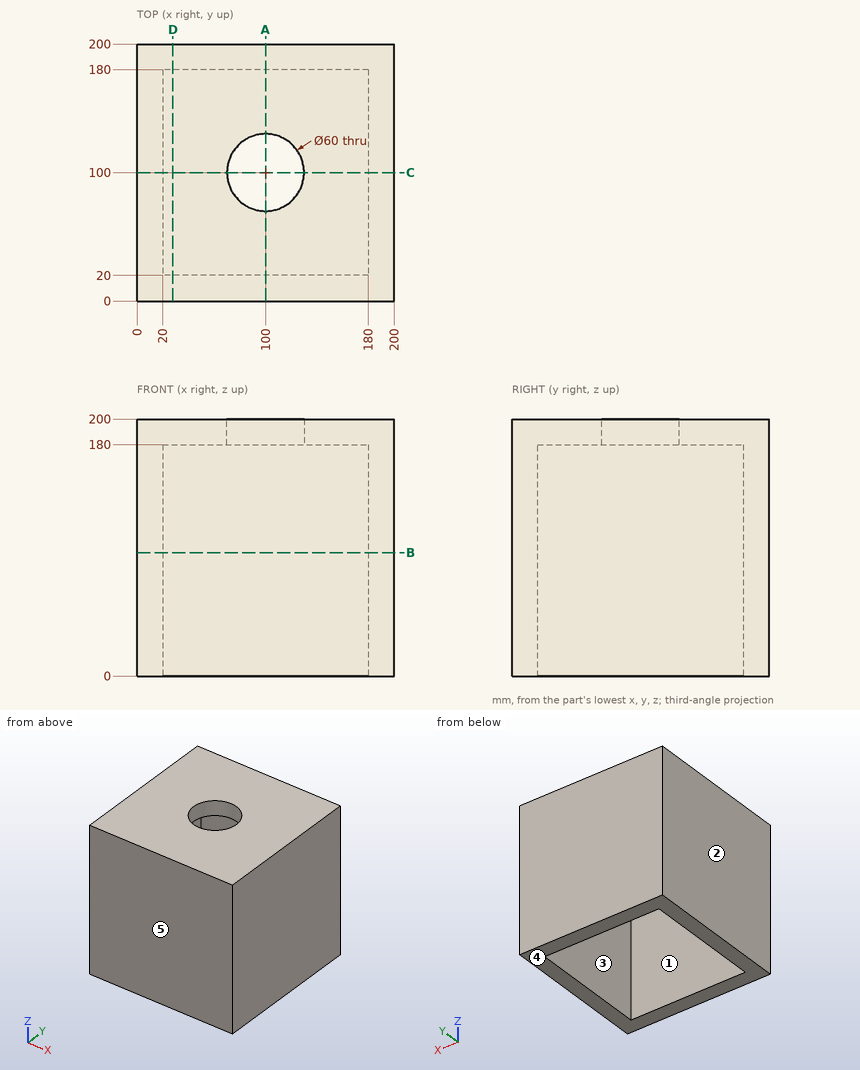
Design review of the part shown in the three views and the two pictorial views. Dimensions are in mm from the part's minimum x, y and z. A direction names the side the tool comes from. Give positions to 0.01 mm unless a question says otherwise; leave off trailing zeros. Write each loop counter-clockwise with the first axis right and the second up, starting at its lowest first coordinate (ties: lowest second). Pieces come first, ordered by that corner, then holes. Notation, with made-up numbers: (-17.75, -18) -> (4.25, -18) arc R27 cw to (4.25, 11) -> close; hole circle Ø8 at (71, 40.5). An arc over 180 degrees is marked (long way). Answer in a Markdown table with one row per item.
1) Clearance check with flat-ended pins moving along their axes: P1, Ø12, axis at x = 78, z = 85.5, coming from the -Y side; P2, Ø1, axis at x = 36.5, y = 177, coming from the -Z side. State where each tip first meets the part, or that it passes through.
Worked answers:
| item | result |
|---|---|
| P1 | y = 0 |
| P2 | z = 180 |
2) Add section B-B on z = 96. State the section outline as (x, y) points.
Worked answers:
| item | result |
|---|---|
| outline | (0, 0) -> (200, 0) -> (200, 200) -> (0, 200) -> close; hole (20, 20) -> (180, 20) -> (180, 180) -> (20, 180) -> close |
3) Mouldability with a two-part tool opening along Y and no side actions: class the marked faces 3, 4 and 5 as +Y half, -Y half, draft (parallel to the pull), parting line (faces both ways), or undercut.
Worked answers:
| item | result |
|---|---|
| face 3 | undercut |
| face 4 | draft |
| face 5 | -Y half |
4) Add section A-A on x = 100. State the section outline as (y, z) points, plus the area to 3 significant figures.
Worked answers:
| item | result |
|---|---|
| outline | (0, 0) -> (20, 0) -> (20, 180) -> (70, 180) -> (70, 200) -> (0, 200) -> close; (130, 180) -> (180, 180) -> (180, 0) -> (200, 0) -> (200, 200) -> (130, 200) -> close |
| area | 10,000 mm² |
5) Add section D-D on x = 28. State the section outline as (y, z) points, plus the area to 3 significant figures.
Worked answers:
| item | result |
|---|---|
| outline | (0, 0) -> (20, 0) -> (20, 180) -> (180, 180) -> (180, 0) -> (200, 0) -> (200, 200) -> (0, 200) -> close |
| area | 11,200 mm² |
6) Tool access review of the marked faces 1 and 2: name each direction out of +Z, -Z, +X, -X, +Y, -Y from which nothing blocks a thin tool from reaching the whole face with its end or side.
Worked answers:
| item | result |
|---|---|
| face 1 | -Z |
| face 2 | +Z, -Z, -X, +Y, -Y |
7) For L1, parallel to Y at x = 130, z = 38; L2, parallel to Y at x = 100, z = 189.5, list the stretches that pass through material, from the lowest coordinate up. Write a range as [from, to].
Worked answers:
| item | result |
|---|---|
| L1 | [0, 20], [180, 200] |
| L2 | [0, 70], [130, 200] |
